Input: part model. Units: mm. Frame: model coordinates. A direction names the side the tool comes from. Round coordinates to 2 decimals unless told otherwise and drop trailing zeros. Loops run counter-clockwise (first coordinate to the right, second up) from the corner with the lowest first, then second, coordinate; pieces in that order, holes last. Notation, with made-up numbers: M -33,11.5 L 13,11.5 A23 cw 13,29.5 Z; hole C -11.75,-29 d9. An arc over 180 degrees is marked long. Return JSON: item names as keys, results as strings. Group by question number.
1) Section B-B (x = -10). Output: boundary loops of the cut face in (y, z) (3 decimals), plus the area to 3 significant figures.
2) Access query for faces 5 (the face through (-31.75, 30, -13)), 6 (the face through (-15.252, 4.819, -3.131)), 7 (the face through (-19, 30, 0)). Directions: +Z, -Z, +X, -X, +Y, -Y. A direction counts if a zero-diameter tool reaches every point of the face in a straight line with its end or side. Return the directions, or none.
3) Mould query, pull axis Y, two halves, no side actions, for faces 1 (the face through (-15.252, 55.619, -3.131)), 2 (the face through (-35.056, 13.766, -6.995)), 3 (the face through (-14, 30, -6.35)), 4 (the face through (-23, 0, -4)). Classes: +Y half, -Y half, draft (parallel to the pull), parting line (faces both ways), or undercut.
4) Material intervals for line 1 (Y direction, x = -6.5, z = -4.75) (3 decimals); line 2 (Y direction, x = -4, z = -5) (3 decimals); line 3 (Z direction, x = -23, y = 43), sorted ascending. Write a range as from..to.
5) Section D-D (y = 39). Output: boundary loops of the cut face in (x, z) (3 decimals), plus the area to 3 significant figures.
6) Section A-A (z = -3.25). Count the separate pieces of the cut face and the enclosed holes in it, plus the area to 3 significant figures.
7) Section C-C (y = 6). Output: boundary loops of the cut face in (x, z) (3 decimals), plus the area to 3 significant figures.
8) Contact query for flat-ended pins moving along their axis: P1, Ø1.5, axis at x = -11.5, y = 31, coming from the -Z side; P2, Ø2, axis at y = 42, z = -8, coming from the +X side; P3, Ø3, axis at y = 32.5, z = -12, coming from the +X side. Output: stop coordinate, or through.
Autodesk Inventor part; units mm, degrees
ref_plane "YZ Plane" through (0, 0, 0) normal (1, 0, 0) x (0, 1, 0)
ref_plane "XZ Plane" through (0, 0, 0) normal (0, 1, 0) x (-1, 0, 0)
ref_plane "XY Plane" through (0, 0, 0) normal (0, 0, 1) x (1, 0, 0)
sketch "Sketch1" plane through (0, 0, 0) normal (0, 1, 0) x (-1, 0, 0)
  line L0 (0, 0) -> (0, -6.35)
  line L1 (0, -6.35) -> (31.75, -6.35)
  line L2 (31.75, -6.35) -> (31.75, -15.875)
  line L3 (31.75, -15.875) -> (38.1, -15.875)
  line L4 (38.1, -15.875) -> (38.1, 0)
  line L5 (38.1, 0) -> (0, 0)
  dimension "d0" = 6.35
  dimension "d1" = 38.1
  dimension "d2" = 15.875
extrude "Extrusion1" add sketch "Sketch1" along normal blind 60.325
sketch "Sketch2" plane through (-38.1, 0, 0) normal (0, 0, 1) x (1, 0, 0)
  line L0 (31.75, 4.7625) -> (31.75, 55.5625) construction
  line L1 (38.1, 0) -> (38.1, 60.325) construction
  line L2 (25.4, 4.7625) -> (31.75, 4.7625) construction
  line L3 (25.4, 2.2098) -> (31.75, 2.2098)
  line L4 (31.75, 7.3152) -> (25.4, 7.3152)
  arc A0 (25.4, 7.3152) -> (25.4, 2.2098) centre (25.4, 4.7625) ccw
  arc A1 (31.75, 2.2098) -> (31.75, 7.3152) centre (31.75, 4.7625) ccw
  line L5 (25.4, 55.5625) -> (31.75, 55.5625) construction
  line L6 (25.4, 53.0098) -> (31.75, 53.0098)
  line L7 (31.75, 58.1152) -> (25.4, 58.1152)
  arc A2 (25.4, 58.1152) -> (25.4, 53.0098) centre (25.4, 55.5625) ccw
  arc A3 (31.75, 53.0098) -> (31.75, 58.1152) centre (31.75, 55.5625) ccw
  point P0 (31.75, 30.1625)
  point P1 (38.1, 30.1625)
  point P2 (28.575, 4.7625)
  point P3 (28.575, 55.5625)
  dimension "d5" = 50.8
  dimension "d6" = 6.35
  dimension "d24" = 5.1054
  dimension "d25" = 6.35
sketch "Sketch3" plane through (-38.1, 0, -15.875) normal (-1, 0, 0) x (0, 0, 1)
  line L0 (7.62, 46.1625) -> (7.62, 14.1625) construction
  line L1 (0, 0) -> (0, 60.325) construction
  line L2 (0, 60.325) -> (15.875, 60.325) construction
  line L3 (15.875, 0) -> (15.875, 60.325) construction
  point P0 (7.62, 30.1625)
  point P1 (0, 30.1625)
  point P2 (7.9375, 60.325)
  dimension "d14" = 32
  dimension "d23" = 8.255
hole "Hole2" at (-38.1, 46.1625, -8.255) at (-38.1, 14.1625, -8.255) direction (1, 0, 0) diameter 2.6416 depth 19.05 tip angle 118
extrude "Extrusion2" cut sketch "Sketch2" against normal blind 25.4
fillet "Fillet2" radius 3.175 1 edges at (-31.75, 30.1625, -6.35)
properties part number "HS-001" material "Aluminum 6061"
Returned:
{
 "1": {"outline": "M 0,-6.35 L 2.21,-6.35 L 2.21,0 L 0,0 Z; M 7.315,-6.35 L 53.01,-6.35 L 53.01,0 L 7.315,0 Z; M 58.115,-6.35 L 60.325,-6.35 L 60.325,0 L 58.115,0 Z", "area": "318 mm^2"},
 "2": {"face 5": "-Z, +X, +Y, -Y", "face 6": "+Z, -Z", "face 7": "+Z, +X, -X, +Y, -Y"},
 "3": {"face 1": "undercut", "face 2": "undercut", "face 3": "draft", "face 4": "-Y half"},
 "4": {"line 1": "y = 0..2.21, 7.315..53.01, 58.115..60.325", "line 2": "y = 0..3.766, 5.759..54.566, 56.559..60.325", "line 3": "z = -6.35..0"},
 "5": {"outline": "M -38.1,-15.875 L -31.75,-15.875 L -31.75,-9.525 A3.175 cw -28.575,-6.35 L 0,-6.35 L 0,0 L -38.1,0 Z", "area": "305 mm^2"},
 "6": {"separate pieces": "1", "enclosed holes": "2", "area": "2,190 mm^2"},
 "7": {"outline": "M -38.1,-15.875 L -31.75,-15.875 L -31.75,-9.525 A3.175 cw -28.575,-6.35 L -14.933,-6.35 L -14.933,0 L -38.1,0 Z; M -4.117,-6.35 L 0,-6.35 L 0,0 L -4.117,0 Z", "area": "236 mm^2"},
 "8": {"P1": "stops at z = -6.35", "P2": "stops at x = -30.5", "P3": "stops at x = -31.75"}
}
